CAD build for the part. Positions are in the model's coordinates, mm. A direction names the side the tool comes from. Give positions to 0.01 mm unless a question says otherwise; leave off trailing zeros. Order: outer loops, then holes, each group sorted by start corner. A loop starts at its lowest first (then second) coordinate and runs counter-clockwise, first axis right, second up.
from build123d import *

# Parameters (mm, degrees)
BOSS_EXTRUDE1_DEPTH = 130
SKETCH2_W           = 3
SKETCH2_H           = 101.039132923
BOSS_EXTRUDE2_DEPTH = 40
SKETCH3_W           = 130
SKETCH3_H           = 101.039132923
BOSS_EXTRUDE3_DEPTH = 3
BOSS_EXTRUDE4_DEPTH = 130
BOSS_EXTRUDE5_DEPTH = 3
BOSS_EXTRUDE6_DEPTH = 3


with BuildPart() as part:
    # Sketch1 → Boss-Extrude1 (new body)
    with BuildSketch(Plane(origin=(0, 0, 0), x_dir=(0, 0, -1), z_dir=(1, 0, 0))):
        with BuildLine():
            Line((0, 0), (0, 108))
            Line((0, 108), (3, 108))
            Line((3, 108), (3, 0))
            ThreePointArc((3, 0), (16.180194847, -31.819805153), (48, -45))
            Line((48, -45), (52.371478475, -48))
            Line((52.371478475, -48), (48, -48))
            ThreePointArc((48, -48), (14.058874503, -33.941125497), (0, 0))
        make_face()
    extrude(amount=BOSS_EXTRUDE1_DEPTH)

    # Sketch2 → Boss-Extrude2 (add)
    with BuildSketch(Plane(origin=(0, 0, -3), x_dir=(-1, 0, 0), z_dir=(0, 0, -1))):
        with Locations((-128.5, 57.480433539)):
            Rectangle(SKETCH2_W, SKETCH2_H)
        with Locations((-1.5, 57.480433539)):
            Rectangle(SKETCH2_W, SKETCH2_H)
    extrude(amount=BOSS_EXTRUDE2_DEPTH)

    # Sketch3 → Boss-Extrude3 (add)
    with BuildSketch(Plane(origin=(0, 0, -43), x_dir=(-1, 0, 0), z_dir=(0, 0, -1))):
        with Locations((-65, 57.480433539)):
            Rectangle(SKETCH3_W, SKETCH3_H)
    extrude(amount=BOSS_EXTRUDE3_DEPTH)

    # Sketch5 → Boss-Extrude4 (add)
    with BuildSketch(Plane(origin=(130, 0, 0), x_dir=(0, 0, -1), z_dir=(1, 0, 0))):
        Polygon((43.040658043, 108), (19.504714564, 148.765449909), (0, 148.765449909), (0, 151.765449909), (20.265766112, 151.765449909), (46, 108), align=None)
    extrude(amount=-BOSS_EXTRUDE4_DEPTH)

    # Sketch6 → Boss-Extrude5 (add)
    with BuildSketch(Plane(origin=(130, 0, 0), x_dir=(0, 0, -1), z_dir=(1, 0, 0))):
        Polygon((43.040658043, 108), (0, 108), (0, 148.765449909), (19.504714564, 148.765449909), align=None)
    extrude(amount=-BOSS_EXTRUDE5_DEPTH)

    # Sketch7 → Boss-Extrude6 (add)
    with BuildSketch(Plane.ZY):
        Polygon((-43.040658043, 108), (0, 108), (0, 148.765449909), (-19.504714564, 148.765449909), align=None)
    extrude(amount=-BOSS_EXTRUDE6_DEPTH)


solid = part.part
1. Saw through at D-D on z = -37. Give the cut face in (x, y), plus the area to 3 significant figures.
2. Saw through at A-A on x = 73.5. Give the cut face in (y, z), plus the area to 3 significant figures.
3. Saw through at C-C on z = -25. Give the cut face in (x, y), plus the area to 3 significant figures.
4. Saw through at B-B on y = 87. Give the cut face in (x, z).
5. Wall check: line 1 (X direction, y = 66, z = -19.5); line 2 (Z direction, x = 30, y = 93); line 3 (Y direction, x = 8, z = -15). Give the ranges that are in metal, low to high.
6. Pin check, flat tips, straight feed: P1, Ø2, axis at y = 23.5, z = -27.5, coming from the -X side; P2, Ø21.5, axis at x = 37.5, z = -19, coming from the -Y side; P3, Ø1, axis at x = 97.5, z = -20.5, coming from the -Y side; P4, Ø1, axis at x = 98.5, z = -28, coming from the +Y side. Stop position of each tip, or through.
7. Mould opens along X. For faces 1 (the flat face through (66, 148.765, -10)), 2 (the flat face through (130, 75, -21)), 3 (the flat face through (65, 6.961, -44)) say: released by +X, released by -X, zero draft, split by the parting line, or undercut.
8. 3-axis set-ups, long thin cutter, end or side, ignore diameter. For faces 4 (the flat face through (65.868, 128.097, -31.437)), 5 (the cylindrical face through (64.09, -31.468, -15.832)), 6 (the flat face through (64, 55, -3)): which of +Z, -Z, +X, -X, +Y, -Y reach the whole face in a straight line?
Reported:
1. outline: (0, -46.72) - (130, -46.72) - (130, -43.63) - (0, -43.63) - close; (0, 6.96) - (3, 6.96) - (3, 118.46) - (127, 118.46) - (127, 6.96) - (130, 6.96) - (130, 123.31) - (0, 123.31) - close
1. area: 1,700 mm2
2. outline: (-48, -52.37) - (-45, -48) arc R45 cw to (0, -3) - (108, -3) - (108, 0) - (0, 0) arc R48 ccw to (-48, -48) - close; (6.96, -46) - (108, -46) - (151.77, -20.27) - (151.77, 0) - (148.77, 0) - (148.77, -19.5) - (108, -43.04) - (108, -43) - (6.96, -43) - close
2. area: 1,030 mm2
3. outline: (0, -42.13) - (130, -42.13) - (130, -38.68) - (0, -38.68) - close; (0, 6.96) - (3, 6.96) - (3, 139.25) - (127, 139.25) - (127, 6.96) - (130, 6.96) - (130, 143.71) - (0, 143.71) - close
3. area: 1,820 mm2
4. outline: (0, -46) - (130, -46) - (130, 0) - (0, 0) - close; hole (3, -43) - (127, -43) - (127, -3) - (3, -3) - close
5. line 1: x = 0 to 3, 127 to 130
5. line 2: z = -46 to -43, -3 to 0
5. line 3: y = -34.86 to -30.59, 148.77 to 151.77
6. P1: stops at x = 0
6. P2: stops at y = -44.4
6. P3: stops at y = -39.69
6. P4: stops at y = 139.46
7. face 1: undercut
7. face 2: released by +X
7. face 3: zero draft
8. face 4: +Z
8. face 5: -Z, +X, -X
8. face 6: none
